The listing builds one solid part. Answer for the finished solid, in the listing's coordinates (mm). A direction names the side the tool comes from. Give positions to 0.01 mm unless a question says otherwise; leave off trailing zeros. Write each loop counter-clockwise with the first axis right and the second up, starting at its lowest first coordinate (ties: lowest second). Pieces come first, ordered by that corner, then holes. Notation, with made-up numbers: (89.5, 28.5) - (103.5, 28.5) arc R5 cw to (103.5, 36.5) - close; hole circle Ø7 at (87, -25). An arc over 180 degrees is marked (long way). Answer in a Markdown table with one row per item. Add a question column.
from build123d import *

# Parameters (mm, degrees)
SKETCH1_W           = 120
SKETCH1_H           = 50
BOSS_EXTRUDE1_DEPTH = 3
SKETCH2_R           = 5
SKETCH2_R_2         = 10
CUT_EXTRUDE1_DEPTH  = 531.57368012


with BuildPart() as part:
    # Sketch1 → Boss-Extrude1 (new body)
    with BuildSketch(Plane.XY):
        with Locations((122.368410373, 32.479010759)):
            Rectangle(SKETCH1_W, SKETCH1_H)
        Polygon((-387.631589627, 7.479010759), (-387.631589627, 57.479010759), (-212.631589627, 154.303594414), (-112.631589627, 154.303594414), (62.368410373, 57.479010759), (62.368410373, 7.479010759), (-112.631589627, 104.303594414), (-212.631589627, 104.303594414), align=None)
        with Locations((-447.631589627, 32.479010759)):
            Rectangle(SKETCH1_W, SKETCH1_H)
    extrude(amount=BOSS_EXTRUDE1_DEPTH)

    # Sketch2 → Cut-Extrude1 (cut, through all)
    with BuildSketch(Plane.XY.offset(3)):
        with Locations((-487.631589627, 17.479010759)):
            Circle(SKETCH2_R)
        with Locations((-407.631589627, 17.479010759)):
            Circle(SKETCH2_R)
        with Locations(Location((82.368410373, 17.479010759, 0), (0, 0, 180))):
            Circle(SKETCH2_R)
        with Locations(Location((162.368410373, 17.479010759, 0), (0, 0, 180))):
            Circle(SKETCH2_R)
        with Locations((-162.631589627, 129.303594414)):
            Circle(SKETCH2_R_2)
    extrude(amount=-CUT_EXTRUDE1_DEPTH, mode=Mode.SUBTRACT)


solid = part.part
1. Section B-B (z = 1.6) is taken. Give the vertices of the cut face in (x, y), and give its area (3 significant figures).
2. A tool of negligible diameter and unlimited length cuts with its end or side. For faces 5 (the face through (-23.907, 55.214, 1.479)), 6 (the face through (-26.36, 106.57, 1.48)), from which of +Z, -Z, +X, -X, +Y, -Y can it reach the whole face along a straight path? Write none if from no direction.
3. Section D-D (x = -258.5) is taken. Give the vertices of the cut face in (y, z).
4. Straight lines are drawn through the part: L1, parallel to X at y = 16, z = 1.4; L2, parallel to Y at x = -129.5, z = 0.3; L3, parallel to X at y = 133.5, z = 1.7. For each, find the intervals that lie inside material, in ascending order. Write a range as [from, to].
5. The mould has two halves that part along X. Classify faces 1 (the face through (-164, 108, 3)), 2 (the face through (-298.907, 56.569, 1.479)), 3 (the face through (-172.622, 129.743, 1.521)), 4 (the face through (-301.36, 105.21, 1.48)): +X half, -X half, draft (parallel to the pull), parting line (faces both ways), or undercut.
6. Section A-A (y = 89) is taken. Give the vertices of the cut face in (x, z).
7. Given pin 1 Ø6 at (x, y) = (-407.63, 17.48) entering from -Z; pin 2 Ø1 at (x, z) = (44, 2) entering from +Y; pin 3 Ø1.5 at (x, z) = (106, 1.5) entering from +Y; pin 4 Ø1.5 at (y, z) = (103, 1.5) entering from -X, each flat-ended and moving along its own axis, determine where each tip first touches the part or whether it passes through.
8. Section C-C (y = 36) is taken. Give the vertices of the cut face in (x, z), and give its area (3 significant figures).
Geometry check:
| question | item | result |
|---|---|---|
| 1 | outline | (-507.63, 7.48) - (-387.63, 7.48) - (-212.63, 104.3) - (-112.63, 104.3) - (62.37, 7.48) - (182.37, 7.48) - (182.37, 57.48) - (62.37, 57.48) - (-112.63, 154.3) - (-212.63, 154.3) - (-387.63, 57.48) - (-507.63, 57.48) - close; hole circle Ø10 at (-487.63, 17.48); hole circle Ø10 at (-407.63, 17.48); hole circle Ø20 at (-162.63, 129.3); hole circle Ø10 at (82.37, 17.48); hole circle Ø10 at (162.37, 17.48) |
| 1 | area | 33,900 mm² |
| 2 | face 5 | +Z, -Z, -Y |
| 2 | face 6 | +Z, -Z, +X, +Y |
| 3 | outline | (78.93, 0) - (128.93, 0) - (128.93, 3) - (78.93, 3) - close |
| 4 | L1 | [-507.63, -492.41], [-482.86, -412.41], [-402.86, -372.23], [46.97, 77.59], [87.14, 157.59], [167.14, 182.37] |
| 4 | L2 | [104.3, 154.3] |
| 4 | L3 | [-250.23, -171.71], [-153.55, -75.03] |
| 5 | face 1 | draft |
| 5 | face 2 | undercut |
| 5 | face 3 | undercut |
| 5 | face 4 | -X half |
| 6 | outline | (-330.66, 0) - (-240.29, 0) - (-240.29, 3) - (-330.66, 3) - close; (-84.97, 0) - (5.4, 0) - (5.4, 3) - (-84.97, 3) - close |
| 7 | pin 1 | through |
| 7 | pin 2 | y = 67.92 |
| 7 | pin 3 | y = 57.48 |
| 7 | pin 4 | x = -306.71 |
| 8 | outline | (-507.63, 0) - (-336.08, 0) - (-336.08, 3) - (-507.63, 3) - close; (10.82, 0) - (182.37, 0) - (182.37, 3) - (10.82, 3) - close |
| 8 | area | 1,030 mm² |
